Geometry: final body of the model. Coordinates: model frame, mm. Face numbers are marked on the shaded views. A direction names the side the tool comes from. Give positions to 0.01 mm unless a question says otherwise; leave off trailing zeros. Write each loop counter-clockwise with the first axis right and the second up, starting at its lowest first coordinate (ties: lowest second). Pieces come first, ordered by that corner, then holes. Notation, with made-up numbers: (47, 7.25) - (74, 7.25) arc R21 cw to (74, 13.25) - close; hole circle Ø7 at (-9, 0.25). An arc over 180 degrees is marked (long way). Return JSON: item names as keys, results as strings.
from build123d import *

# Parameters (mm, degrees)
SKETCH1_W           = 10.5
SKETCH1_H           = 5
BOSS_EXTRUDE1_DEPTH = 5.5
SKETCH2_W           = 6.1
SKETCH2_H           = 3
CUT_EXTRUDE1_DEPTH  = 0.5
SKETCH3_W           = 3
SKETCH3_H           = 3
BOSS_EXTRUDE2_DEPTH = 5
BOSS_EXTRUDE3_DEPTH = 0.4
LPATTERN1_COUNT     = 2
LPATTERN1_PITCH     = 3
LPATTERN1_COL_COUNT = 2
LPATTERN1_COL_PITCH = 3


with BuildPart() as part:
    # Sketch1 → Boss-Extrude1 (new body)
    with BuildSketch(Plane.XY):
        with Locations((0, 2.5)):
            Rectangle(SKETCH1_W, SKETCH1_H)
    extrude(amount=BOSS_EXTRUDE1_DEPTH)

    # Sketch2 → Cut-Extrude1 (cut)
    with BuildSketch(Plane(origin=(0, 5, 0), x_dir=(1, 0, 0), z_dir=(0, 1, 0))):
        with Locations((0, -2.75)):
            Rectangle(SKETCH2_W, SKETCH2_H)
    extrude(amount=-CUT_EXTRUDE1_DEPTH, mode=Mode.SUBTRACT)

    # Sketch3 → Boss-Extrude2 (add)
    with BuildSketch(Plane(origin=(0, 4.5, 0), x_dir=(1, 0, 0), z_dir=(0, 1, 0))):
        with Locations((1.55, -2.75)):
            Rectangle(SKETCH3_W, SKETCH3_H)
    extrude(amount=BOSS_EXTRUDE2_DEPTH)

    # Sketch4 → Boss-Extrude3 (add, symmetric)
    with BuildSketch(Plane(origin=(0, 0, 0), x_dir=(0, 0, -1), z_dir=(1, 0, 0))):
        with BuildLine():
            Line((-2.5, 0), (-2.5, -0.65))
            ThreePointArc((-2.5, -0.65), (-2.324264069, -1.074264069), (-1.9, -1.25))
            Line((-1.9, -1.25), (2.5, -1.25))
            Line((2.5, -1.25), (2.5, -1.75))
            Line((2.5, -1.75), (-1.9, -1.75))
            ThreePointArc((-1.9, -1.75), (-2.677817459, -1.427817459), (-3, -0.65))
            Line((-3, -0.65), (-3, 0))
            Line((-3, 0), (-2.5, 0))
        make_face()
    boss_extrude3 = extrude(amount=BOSS_EXTRUDE3_DEPTH, both=True)

    # LPattern1: Boss-Extrude3 ×2
    with Locations(*[(-i * LPATTERN1_PITCH, 0, 0) for i in range(1, LPATTERN1_COUNT)]):
        add(boss_extrude3)

    # LPattern1 col: Boss-Extrude3 ×2
    with Locations(*[(i * LPATTERN1_COL_PITCH, 0, 0) for i in range(1, LPATTERN1_COL_COUNT)]):
        add(boss_extrude3)


solid = part.part
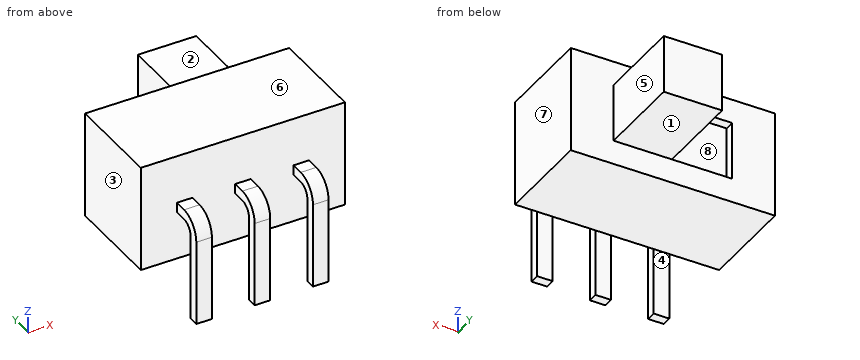
Q1. Pin query (flat end, axial travel): P1, Ø1.5, axis at x = -3, y = 6.5, coming from the +Z side; P2, Ø5.5, axis at x = 1, y = 1.5, coming from the -Z side; P3, Ø1.9, axis at y = -1, z = 1.5, coming from the +X side; P4, Ø3, axis at x = 1, z = 0.5, coming from the +Y side. Return the tip coordinate at first contact, or that it passes through.
Answer key:
{"P1": "passes through", "P2": "stops at z = 0", "P3": "stops at x = 3.4", "P4": "stops at y = 9.5"}
Q2. Section query D-D, the plane x = -2. Return the cut outline in (y, z), plus the area to 3 significant figures.
Answer key:
{"outline": "(0, 0) - (5, 0) - (5, 1.25) - (4.5, 1.25) - (4.5, 4.25) - (5, 4.25) - (5, 5.5) - (0, 5.5) - close", "area": "26.0 mm^2"}
Q3. Section query B-B, the plane y = -0.5. Return the cut outline in (x, z).
Answer key:
{"outline": "(-3.4, 2.5) - (-2.6, 2.5) - (-2.6, 3) - (-3.4, 3) - close; (-0.4, 2.5) - (0.4, 2.5) - (0.4, 3) - (-0.4, 3) - close; (2.6, 2.5) - (3.4, 2.5) - (3.4, 3) - (2.6, 3) - close"}
Q4. Mould query, pull axis X, two halves, no side actions, for the marked faces 6, 7 and 8. Classes: pulls with the +X half, pulls with the -X half, needs draft (parallel to the pull), parting line crosses it, or undercut.
Answer key:
{"face 6": "needs draft", "face 7": "pulls with the +X half", "face 8": "undercut"}
Q5. Section query C-C, the plane z = -1. Return the cut outline in (x, y).
Answer key:
{"outline": "(-3.4, -1.75) - (-2.6, -1.75) - (-2.6, -1.25) - (-3.4, -1.25) - close; (-0.4, -1.75) - (0.4, -1.75) - (0.4, -1.25) - (-0.4, -1.25) - close; (2.6, -1.75) - (3.4, -1.75) - (3.4, -1.25) - (2.6, -1.25) - close"}
Q6. Section query A-A, the plane z = 1.5. Return the cut outline in (x, y).
Answer key:
{"outline": "(-5.25, 0) - (5.25, 0) - (5.25, 5) - (3.05, 5) - (3.05, 9.5) - (0.05, 9.5) - (0.05, 4.5) - (-3.05, 4.5) - (-3.05, 5) - (-5.25, 5) - close; (-3.4, -1.75) - (-2.6, -1.75) - (-2.6, -1.25) - (-3.4, -1.25) - close; (-0.4, -1.75) - (0.4, -1.75) - (0.4, -1.25) - (-0.4, -1.25) - close; (2.6, -1.75) - (3.4, -1.75) - (3.4, -1.25) - (2.6, -1.25) - close"}
Q7. Material intervals for probe 1 along Z at (x, y) = (2, 7.25); probe 2 along Y at (x, z) = (-3.75, 4.5); probe 3 along Y at (x, z) = (-3, -1), sorted ascending. Write a range as [from, to].
Answer key:
{"probe 1": "z = [1.25, 4.25]", "probe 2": "y = [0, 5]", "probe 3": "y = [-1.75, -1.25]"}
Q8. Set-up query: the marked faces 1, 2, 3, 4 and 5. Return all of +Z, -Z, +X, -X, +Y, -Y with unobstructed straight access to the full face (end or side cutting, diameter ignored); none if empty.
Answer key:
{"face 1": "-Z, +X, -X, +Y", "face 2": "+Z, +X, -X, +Y", "face 3": "+Z, -Z, -X, +Y, -Y", "face 4": "-Z, +X, -X", "face 5": "+Z, -Z, +X, +Y"}
